CAD build for the part. Positions are in the model's coordinates, mm. A direction names the side the tool comes from. Coordinates: 2 decimals unless noted, no trailing zeros. Write each loop counter-clockwise with the first axis right and the second up, starting at its lowest first coordinate (ties: lowest second). Pieces come first, ordered by that corner, then holes. Notation, with made-up numbers: M -6,2.25 L 31,2.25 A13 ccw 31,6.25 Z; hole C 82,-17 d10. An arc over 180 degrees is marked long. Put each result on its own line as item: value. Start each with the question number.
```python
from build123d import *

# Parameters (mm, degrees)
SKETCH1_R                = 6.985
BLANK_DISK_DEPTH         = 2
GEAR_TOOTH_CUT_DEPTH     = 11.657412937
GEAR_START               = -2.000000064
GEAR_TEETH_REVOLVE_DEPTH = 4.000000128


# Read off the part's stored shape, not the designer's step: GEAR TEETH REVOLVE
with BuildPart() as part:
    # Sketch1 → BLANK DISK (new, symmetric)
    with BuildSketch(Plane.XY):
        Circle(SKETCH1_R)
    extrude(amount=BLANK_DISK_DEPTH, both=True)

    # Sketch2 → GEAR TOOTH CUT (cut, through all)
    with BuildSketch(Plane.XY.offset(2.000000064)):
        with BuildLine():
            ThreePointArc((-5.763009467, -3.946890786), (-6.563752956, -2.389010701), (-6.951733872, -0.680897326))
            ThreePointArc((-6.951733872, -0.680897326), (-6.303106227, -0.89616004), (-5.627259472, -0.997585))
            ThreePointArc((-5.627259472, -0.997585), (-5.00805343, -1.01182167), (-4.389706578, -0.976241119))
            ThreePointArc((-4.389706578, -0.976241119), (-4.103194142, -1.046520353), (-3.923782009, -1.280699416))
            ThreePointArc((-3.923782009, -1.280699416), (-3.878581292, -1.411688142), (-3.82900912, -1.541085788))
            ThreePointArc((-3.82900912, -1.541085788), (-3.815919388, -1.835801253), (-3.990226026, -2.073804914))
            ThreePointArc((-3.990226026, -2.073804914), (-4.486777934, -2.444014326), (-4.951966126, -2.852938219))
            ThreePointArc((-4.951966126, -2.852938219), (-5.404500069, -3.365060167), (-5.763009467, -3.946890786))
        make_face()
    extrude(amount=-GEAR_TOOTH_CUT_DEPTH, mode=Mode.SUBTRACT)

    # GEAR TEETH REVOLVE outline → GEAR TEETH REVOLVE (cut)
    with BuildSketch(Plane.XY.offset(GEAR_START)):
        with BuildLine():
            ThreePointArc((-4.887664738, -4.990086011), (-3.4925, -6.049187445), (-1.877708884, -6.727884834))
            ThreePointArc((-1.877708884, -6.727884834), (-1.977068265, -6.051731323), (-1.959592795, -5.368539939))
            ThreePointArc((-1.959592795, -5.368539939), (-1.866089177, -4.756268856), (-1.723674371, -4.15349458))
            ThreePointArc((-1.723674371, -4.15349458), (-1.743133543, -3.859131051), (-1.942600309, -3.641779824))
            ThreePointArc((-1.942600309, -3.641779824), (-2.06375, -3.574519854), (-2.182573688, -3.503231129))
            ThreePointArc((-2.182573688, -3.503231129), (-2.470538755, -3.439163456), (-2.735194635, -3.569493083))
            ThreePointArc((-2.735194635, -3.569493083), (-3.186005068, -3.994215061), (-3.669495571, -4.381327111))
            ThreePointArc((-3.669495571, -4.381327111), (-4.25241893, -4.738057004), (-4.887664738, -4.990086011))
        make_face()
        with BuildLine():
            ThreePointArc((-0.536602953, -6.964357994), (1.212932521, -6.878882154), (2.886192555, -6.360826796))
            ThreePointArc((2.886192555, -6.360826796), (2.375455753, -5.906730136), (1.949695784, -5.372142157))
            ThreePointArc((1.949695784, -5.372142157), (1.627763445, -4.843012329), (1.34940368, -4.289717971))
            ThreePointArc((1.34940368, -4.289717971), (1.14528386, -4.07673054), (0.852772776, -4.038444607))
            ThreePointArc((0.852772776, -4.038444607), (0.716732854, -4.064794001), (0.579885119, -4.086562064))
            ThreePointArc((0.579885119, -4.086562064), (0.318109172, -4.222583755), (0.199145275, -4.492539562))
            ThreePointArc((0.199145275, -4.492539562), (0.126810473, -5.107670834), (0.00526609, -5.714997574))
            ThreePointArc((0.00526609, -5.714997574), (-0.211977555, -6.362964438), (-0.536602953, -6.964357994))
        make_face()
        with BuildLine():
            ThreePointArc((4.065541317, -5.67992947), (5.350820435, -4.489871453), (6.29961242, -3.017467208))
            ThreePointArc((6.29961242, -3.017467208), (5.616477625, -2.997904272), (4.946700037, -2.862059354))
            ThreePointArc((4.946700037, -2.862059354), (4.35996746, -2.663656509), (3.791080751, -2.418734649))
            ThreePointArc((3.791080751, -2.418734649), (3.497810216, -2.386782502), (3.249124002, -2.545476276))
            ThreePointArc((3.249124002, -2.545476276), (3.161848439, -2.653105859), (3.071009233, -2.757745191))
            ThreePointArc((3.071009233, -2.757745191), (2.957910282, -3.030210187), (3.040302898, -3.313476852))
            ThreePointArc((3.040302898, -3.313476852), (3.380289985, -3.831190659), (3.677563689, -4.374557157))
            ThreePointArc((3.677563689, -4.374557157), (3.927650474, -5.010570096), (4.065541317, -5.67992947))
        make_face()
        with BuildLine():
            ThreePointArc((6.765373622, -1.737798823), (6.985, 0), (6.765373622, 1.737798823))
            ThreePointArc((6.765373622, 1.737798823), (6.229487195, 1.313674319), (5.629088366, 0.987212828))
            ThreePointArc((5.629088366, 0.987212828), (5.052094245, 0.762053795), (4.458869006, 0.584001497))
            ThreePointArc((4.458869006, 0.584001497), (4.213672298, 0.419967595), (4.125173997, 0.138548695))
            ThreePointArc((4.125173997, 0.138548695), (4.1275, 0), (4.125173997, -0.138548695))
            ThreePointArc((4.125173997, -0.138548695), (4.213672298, -0.419967595), (4.458869006, -0.584001497))
            ThreePointArc((4.458869006, -0.584001497), (5.052094245, -0.762053795), (5.629088366, -0.987212828))
            ThreePointArc((5.629088366, -0.987212828), (6.229487195, -1.313674319), (6.765373622, -1.737798823))
        make_face()
        with BuildLine():
            ThreePointArc((6.29961242, 3.017467208), (5.350820435, 4.489871453), (4.065541318, 5.679929471))
            ThreePointArc((4.065541318, 5.679929471), (3.927650474, 5.010570096), (3.677563689, 4.374557157))
            ThreePointArc((3.677563689, 4.374557157), (3.380289985, 3.831190659), (3.040302898, 3.313476852))
            ThreePointArc((3.040302898, 3.313476852), (2.957910282, 3.030210187), (3.071009233, 2.757745191))
            ThreePointArc((3.071009233, 2.757745191), (3.161848439, 2.653105859), (3.249124002, 2.545476276))
            ThreePointArc((3.249124002, 2.545476276), (3.497810216, 2.386782502), (3.791080751, 2.418734649))
            ThreePointArc((3.791080751, 2.418734649), (4.35996746, 2.663656509), (4.946700037, 2.862059354))
            ThreePointArc((4.946700037, 2.862059354), (5.616477625, 2.997904272), (6.29961242, 3.017467208))
        make_face()
        with BuildLine():
            ThreePointArc((2.886192555, 6.360826797), (1.212932521, 6.878882155), (-0.536602953, 6.964357994))
            ThreePointArc((-0.536602953, 6.964357994), (-0.211977555, 6.362964438), (0.00526609, 5.714997574))
            ThreePointArc((0.00526609, 5.714997574), (0.126810473, 5.107670834), (0.199145275, 4.492539562))
            ThreePointArc((0.199145275, 4.492539562), (0.318109172, 4.222583755), (0.579885119, 4.086562064))
            ThreePointArc((0.579885119, 4.086562064), (0.716732854, 4.064794001), (0.852772776, 4.038444607))
            ThreePointArc((0.852772776, 4.038444607), (1.14528386, 4.07673054), (1.34940368, 4.289717971))
            ThreePointArc((1.34940368, 4.289717971), (1.627763445, 4.843012329), (1.949695784, 5.372142157))
            ThreePointArc((1.949695784, 5.372142157), (2.375455753, 5.906730136), (2.886192555, 6.360826797))
        make_face()
        with BuildLine():
            ThreePointArc((-1.877708884, 6.727884835), (-3.4925, 6.049187445), (-4.887664739, 4.990086012))
            ThreePointArc((-4.887664739, 4.990086012), (-4.25241893, 4.738057004), (-3.669495571, 4.381327111))
            ThreePointArc((-3.669495571, 4.381327111), (-3.186005068, 3.994215061), (-2.735194635, 3.569493083))
            ThreePointArc((-2.735194635, 3.569493083), (-2.470538755, 3.439163456), (-2.182573688, 3.503231129))
            ThreePointArc((-2.182573688, 3.503231129), (-2.06375, 3.574519854), (-1.942600309, 3.641779824))
            ThreePointArc((-1.942600309, 3.641779824), (-1.743133543, 3.859131051), (-1.723674371, 4.15349458))
            ThreePointArc((-1.723674371, 4.15349458), (-1.866089177, 4.756268856), (-1.959592795, 5.368539939))
            ThreePointArc((-1.959592795, 5.368539939), (-1.977068265, 6.051731323), (-1.877708884, 6.727884835))
        make_face()
        with BuildLine():
            ThreePointArc((-3.923782009, 1.280699416), (-3.878581292, 1.411688142), (-3.82900912, 1.541085788))
            ThreePointArc((-3.82900912, 1.541085788), (-3.815919388, 1.835801253), (-3.990226026, 2.073804914))
            ThreePointArc((-3.990226026, 2.073804914), (-4.486777933, 2.444014326), (-4.951966126, 2.852938219))
            ThreePointArc((-4.951966126, 2.852938219), (-5.404500069, 3.365060167), (-5.763009467, 3.946890786))
            ThreePointArc((-5.763009467, 3.946890786), (-6.563752956, 2.389010701), (-6.951733872, 0.680897326))
            ThreePointArc((-6.951733872, 0.680897326), (-6.303106227, 0.89616004), (-5.627259472, 0.997585))
            ThreePointArc((-5.627259472, 0.997585), (-5.00805343, 1.01182167), (-4.389706578, 0.976241119))
            ThreePointArc((-4.389706578, 0.976241119), (-4.103194142, 1.046520353), (-3.923782009, 1.280699416))
        make_face()
    extrude(amount=GEAR_TEETH_REVOLVE_DEPTH, mode=Mode.SUBTRACT)


solid = part.part
```
(1) Drop flat-ended pins along their axis: pin 1 (2 mm diameter, centred on y = 3, z = -0.5, fed in from +X); pin 2 (2 mm diameter, centred on y = 3.5, z = 1.5, fed in from +X); pin 3 (1 mm diameter, centred on x = -4.5, z = 1, fed in from -Y). Give the stop position or say it passes through.
(2) Slice it at D-D, the plane x = 2.5. Write the cut outline in (y, z).
(3) Drill centre lines: line 1 (X direction, y = 4.5, z = -1.2); line 2 (Y direction, x = -4, z = 0.75); line 3 (Y direction, x = 1, z = -0.6). Where is each one in solid material? Low to high. Write a range as [from, to].
(4) Slice it at A-A, the plane x = 5.25. Write the cut outline in (y, z), then the cut area to 3 significant figures.
(5) Slice it at C-C, the plane x = -2.5. Write the cut outline in (y, z), then the cut area to 3 significant figures.
(6) Slice it at B-B, the plane y = -6. Write the cut outline in (x, z), then the cut area to 3 significant figures.
(7) Which spindle directions (+Z, -Z, +X, -X, +Y, -Y) get a long thin tool onto all of the face, cutting with end or side? Do faces 1 (the face through (2.38, -5.91, -0.03)), 2 (the face through (4.35, 2.66, -0.03)), 3 (the face through (2.37, 5.9, -0.03)). Say none if no direction does.
(8) Two-plate mould, pull along Y, no slides. Class faces 4 (the face through (-1.978, 6.042, -0.028)), 5 (the face through (0, 0, -2)), 6 (the face through (-1.222, -6.877, 0.028)), 7 (the face through (5.06, 0.765, -0.028)): +Y half, -Y half, draft (parallel to the pull), parting line (faces both ways), or undercut.
Result set:
1. pin 1: stops at x = 6.69
1. pin 2: stops at x = 6.52
1. pin 3: stops at y = -4.99
2. outline: M -6.03,-2 L 6.03,-2 L 6.03,2 L -6.03,2 Z
3. line 1: x = [-5.34, -3.84], [-1.81, 0.2], [1.45, 3.74]
3. line 2: y = [-4.6, -2.08], [-1.14, 1.14], [2.08, 4.6]
3. line 3: y = [-4.03, 4.03]
4. outline: M -2.94,-2 L -0.83,-2 L -0.83,2 L -2.94,2 Z; M 0.83,-2 L 2.94,-2 L 2.94,2 L 0.83,2 Z
4. area: 16.8 mm^2
5. outline: M -3.44,-2 L 3.44,-2 L 3.44,2 L -3.44,2 Z
5. area: 27.5 mm^2
6. outline: M -1.98,-2 L -0.08,-2 L -0.08,2 L -1.98,2 Z; M 2.47,-2 L 3.58,-2 L 3.58,2 L 2.47,2 Z
6. area: 12.1 mm^2
7. face 1: +Z, -Z, -Y
7. face 2: +Z, -Z
7. face 3: +Z, -Z, +Y
8. face 4: undercut
8. face 5: draft
8. face 6: -Y half
8. face 7: undercut
